For this review, take the finished solid that the model builds, in its own axes (mm). A direction names the side the tool comes from. Coordinates: 2 decimals unless noted, no trailing zeros. Write each loop counter-clockwise with the first axis right and the second up, starting at its lowest first coordinate (ties: lowest second). Pieces come first, ordered by that corner, then holes.
1) Mouldability with a two-part tool opening along Z and no side actions: class faces 1 (the face through (8, -77, -16.606)), 2 (the face through (-57.78, -25.04, 3.93)), 3 (the face through (7, 0, -16)) as pulls with the +Z half, pulls with the -Z half, needs draft (parallel to the pull), parting line crosses it, or undercut.
2) For faces 4 (the face through (86, -25.4, -42)), 5 (the face through (7, -50.8, 9)), 6 (the face through (-44.113, -64, -42)), list the 3-axis set-ups (+Z, -Z, +X, -X, +Y, -Y) from which the entire face can be reached by the end or side of a thin tool; tool diameter is ignored.
3) We need section B-B on z = 16. Write out the cut boundary in (x, y).
4) We need section A-A on y = -16. Write out the cut boundary in (x, z).
5) We need section D-D on z = -39. Write out the cut boundary in (x, y).
6) We need section C-C on x = 44. Write out the cut boundary in (y, z).
7) To check wall thickness, follow line 1 along X through (y, z) = (-37.5, 9); line 2 along X through (y, z) = (-35.5, 11); line 3 along X through (y, z) = (-94, -30.5). State the ranges of each line that lie inside material, in increasing order.
8) Insertion check: P1, Ø15, axis at y = -68.5, z = -30.5, coming from the +X side; P2, Ø12, axis at y = -36.5, z = -55, coming from the -X side; P3, Ø4, axis at x = -40, z = -49.5, coming from the +Y side; P4, Ø15, axis at x = -69.51, z = 8.79, coming from the +Y side. Each pin has a flat end and moves straight along its axis. Give the tip position at first contact, or say it passes through.
from build123d import *

# Parameters (mm, degrees)
F0_R     = 12.7
F1_DEPTH = 101.6
F2_W     = 50.8
F2_H     = 50.8
F3_DEPTH = 76.2
F4_W     = 180.9563313782
F4_H     = 50.8
F5_DEPTH = 50.8
F6_W     = 50.8
F6_H     = 50.8
F7_DEPTH = 203.2


with BuildPart() as f1:
    # F0 (on Front) → F1 (new body)
    with BuildSketch(Plane.XZ):
        with BuildLine():
            Line((86.0436633229, 34.1943300605), (-69.5126680553, 34.1943300605))
            ThreePointArc((-69.5126680553, 34.1943300605), (-87.4731802974, 26.7548423026), (-94.9126680553, 8.7943300605))
            Line((-94.9126680553, 8.7943300605), (-94.9126680553, -67.4056699395))
            Line((-94.9126680553, -67.4056699395), (111.4436633229, -67.4056699395))
            Line((111.4436633229, -67.4056699395), (111.4436633229, 8.7943300605))
            ThreePointArc((111.4436633229, 8.7943300605), (104.0041755651, 26.7548423026), (86.0436633229, 34.1943300605))
        make_face()
        with Locations((-69.5126680553, 8.7943300605)):
            Circle(F0_R, mode=Mode.SUBTRACT)
        with Locations((86.0436633229, 8.7943300605)):
            Circle(F0_R, mode=Mode.SUBTRACT)
    extrude(amount=F1_DEPTH)

    # F2 (on face) → F3 (cut)
    with BuildSketch(Plane.XZ.offset(101.6)):
        with Locations((-69.5126680553, -42.0056699395)):
            Rectangle(F2_W, F2_H)
        with Locations((86.0436633229, -42.0056699395)):
            Rectangle(F2_W, F2_H)
    extrude(amount=-F3_DEPTH, mode=Mode.SUBTRACT)

    # F4 (on face) → F5 (cut)
    with BuildSketch(Plane.XZ.offset(101.6)):
        with Locations((20.9654976338, 8.7943300605)):
            Rectangle(F4_W, F4_H)
    extrude(amount=-F5_DEPTH, mode=Mode.SUBTRACT)

    # F6 (on face) → F7 (cut)
    with BuildSketch(Plane.YZ.offset(-69.5126680553)):
        with Locations((-76.2, 8.7943300605)):
            Rectangle(F6_W, F6_H)
    extrude(amount=-F7_DEPTH, mode=Mode.SUBTRACT)


solid = f1.part
Result:
1. face 1: pulls with the +Z half
1. face 2: undercut
1. face 3: needs draft
2. face 4: -Z, +X, -Y
2. face 5: +Z, +X, -X, -Y
2. face 6: -Z, -X, -Y
3. outline: (-93.87, -50.8) - (-79.97, -50.8) - (-79.97, 0) - (-93.87, 0) - close; (-59.05, -50.8) - (75.59, -50.8) - (75.59, 0) - (-59.05, 0) - close; (96.5, -50.8) - (110.4, -50.8) - (110.4, 0) - (96.5, 0) - close
4. outline: (-94.91, -67.41) - (111.44, -67.41) - (111.44, 8.79) arc R25.4 ccw to (86.04, 34.19) - (-69.51, 34.19) arc R25.4 ccw to (-94.91, 8.79) - close; hole circle Ø25.4 at (-69.51, 8.79); hole circle Ø25.4 at (86.04, 8.79)
5. outline: (-94.91, -25.4) - (-44.11, -25.4) - (-44.11, -101.6) - (60.64, -101.6) - (60.64, -25.4) - (111.44, -25.4) - (111.44, 0) - (-94.91, 0) - close
6. outline: (-101.6, -67.41) - (0, -67.41) - (0, 34.19) - (-50.8, 34.19) - (-50.8, -16.61) - (-101.6, -16.61) - close
7. line 1: x = -94.91 to -82.21, -56.81 to 73.35, 98.74 to 111.44
7. line 2: x = -94.82 to -82.02, -57.01 to 73.54, 98.55 to 111.35
7. line 3: x = -44.11 to 60.64
8. P1: stops at x = 60.64
8. P2: stops at x = -44.11
8. P3: stops at y = 0
8. P4: passes through
